from build123d import *

# Parameters (mm, degrees)
BOSS_EXTRUDE1_DEPTH      = 55
BOSS_EXTRUDE2_DEPTH      = 25
BOSS_EXTRUDE2_DEPTH_BACK = 25
SKETCH3_W                = 38.273351984
SKETCH3_H                = 18.275853279


with BuildPart() as part:
    # Sketch1 → Boss-Extrude1 (new body)
    with BuildSketch(Plane(origin=(0, 0, 0), x_dir=(1, 0, 0), z_dir=(0, 1, 0))):
        Polygon((87.5, -31.724146721), (87.5, 31.724146721), (49.226648016, 31.724146721), (49.226648016, 50), (-49.226648016, 50), (-49.226648016, 31.724146721), (-87.5, 31.724146721), (-87.5, -31.724146721), (-49.226648016, -31.724146721), (-49.226648016, -50), (49.226648016, -50), (49.226648016, -31.724146721), align=None)
    extrude(amount=BOSS_EXTRUDE1_DEPTH)

    # Sketch3 → Boss-Extrude2 (add, two sides: drawn at the far end of the back side and taken through both)
    with BuildSketch(Plane(origin=(0, 55, 0), x_dir=(1, 0, 0), z_dir=(0, 1, 0)).offset(-BOSS_EXTRUDE2_DEPTH_BACK)):
        with Locations((-68.363324008, 40.86207336)):
            Rectangle(SKETCH3_W, SKETCH3_H)
        with Locations((-68.363324008, -40.86207336)):
            Rectangle(SKETCH3_W, SKETCH3_H)
        with Locations((68.363324008, -40.86207336)):
            Rectangle(SKETCH3_W, SKETCH3_H)
        with Locations((68.363324008, 40.86207336)):
            Rectangle(SKETCH3_W, SKETCH3_H)
    extrude(amount=BOSS_EXTRUDE2_DEPTH + BOSS_EXTRUDE2_DEPTH_BACK)


solid = part.part
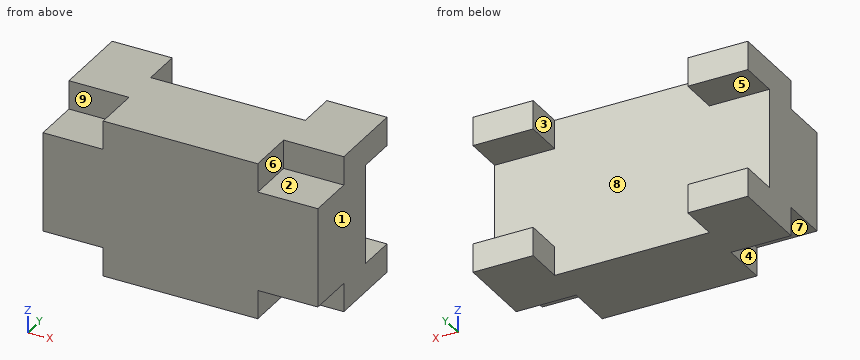
Geometry: final body of the model. Coordinates: model frame, mm. Face numbers are marked on the shaded views. A direction names the side the tool comes from. Give positions to 0.01 mm unless a question says otherwise; leave off trailing zeros. Write each loop counter-clockwise with the first axis right and the second up, starting at its lowest first coordinate (ties: lowest second). Pieces come first, ordered by that corner, then holes. Notation, with made-up numbers: (-37.75, 10.5) -> (1.25, 10.5) arc R16 ccw to (1.25, 35.5) -> close; hole circle Ø8 at (15, -7.75). An arc over 180 degrees is marked (long way). Answer in a Markdown table with one row per item.
(1) Section query A-A on y = 73. Return loops of the section in (x, z).
Answers below:
| item | result |
|---|---|
| outline | (-87.5, -50) -> (-49.23, -50) -> (-49.23, -31.72) -> (-87.5, -31.72) -> close; (-87.5, 31.72) -> (-49.23, 31.72) -> (-49.23, 50) -> (-87.5, 50) -> close; (49.23, -50) -> (87.5, -50) -> (87.5, -31.72) -> (49.23, -31.72) -> close; (49.23, 31.72) -> (87.5, 31.72) -> (87.5, 50) -> (49.23, 50) -> close |
(2) Section query C-C on x = 72. Return loops of the section in (y, z).
Answers below:
| item | result |
|---|---|
| outline | (0, -31.72) -> (30, -31.72) -> (30, -50) -> (80, -50) -> (80, -31.72) -> (55, -31.72) -> (55, 31.72) -> (80, 31.72) -> (80, 50) -> (30, 50) -> (30, 31.72) -> (0, 31.72) -> close |
(3) Set-up query: the marked faces 5, 6, 7, 8 and 9. Return all of +Z, -Z, +X, -X, +Y, -Y with unobstructed straight access to the full face (end or side cutting, diameter ignored); none if empty.
Answers below:
| item | result |
|---|---|
| face 5 | +X, -X, +Y |
| face 6 | +Z, +X, -Y |
| face 7 | -Z, -X, -Y |
| face 8 | +Y |
| face 9 | +Z, -X, -Y |
(4) Ray query, line 1 along Z through (x, y) = (65, 75.5); line 2 along Y through (x, z) = (38, 36.5); line 3 along Z through (x, y) = (66, 22). Return the intervals inside material, ascending. Write a range as [from, to].
Answers below:
| item | result |
|---|---|
| line 1 | [-50, -31.72], [31.72, 50] |
| line 2 | [0, 55] |
| line 3 | [-31.72, 31.72] |
(5) Section query B-B on y = 13.5. Return loops of the section in (x, z).
Answers below:
| item | result |
|---|---|
| outline | (-87.5, -31.72) -> (-49.23, -31.72) -> (-49.23, -50) -> (49.23, -50) -> (49.23, -31.72) -> (87.5, -31.72) -> (87.5, 31.72) -> (49.23, 31.72) -> (49.23, 50) -> (-49.23, 50) -> (-49.23, 31.72) -> (-87.5, 31.72) -> close |
(6) Draft query along X for the marked faces 1, 2, 3 and 4. Return one class per face: +X half, -X half, draft (parallel to the pull), parting line (faces both ways), or undercut.
Answers below:
| item | result |
|---|---|
| face 1 | +X half |
| face 2 | draft |
| face 3 | undercut |
| face 4 | -X half |
(7) Section query D-D on z = 1. Return loops of the section in (x, y).
Answers below:
| item | result |
|---|---|
| outline | (-87.5, 0) -> (87.5, 0) -> (87.5, 55) -> (-87.5, 55) -> close |
(8) Pin query (flat end, axial travel): pin 1 (5.5 mm diameter, centred on y = 12, z = 37.5, fed in from +X); pin 2 (14.5 mm diameter, centred on y = 8.5, z = 41, fed in from -X); pin 3 (2 mm diameter, centred on x = 20.5, z = -19, fed in from +Y). Return the tip coordinate at first contact, or that it passes through.
Answers below:
| item | result |
|---|---|
| pin 1 | x = 49.23 |
| pin 2 | x = -49.23 |
| pin 3 | y = 55 |
